The listing builds one solid part. Answer for the finished solid, in the listing's coordinates (mm). Face numbers are marked on the shaded views. A direction names the side the tool comes from. Round coordinates to 2 decimals unless told otherwise and drop trailing zeros. Write each loop counter-clockwise with the first axis right and the second up, starting at its lowest first coordinate (ties: lowest second). Pieces come first, ordered by that corner, then holes.
(1) Each of these flat-tipped pins is pushed along its axis until it touches: pin 1 Ø3.5 at (y, z) = (14, 1) entering from +X; pin 2 Ø3.5 at (y, z) = (-2, 1) entering from -X; pin 3 Ø3 at (y, z) = (8, 10.5) entering from -X; pin 4 Ø5 at (x, y) = (0, 8.5) entering from -Z. Where does it stop, or does it pass through?
(2) For the marked faces 1 and 2, determine the directions among +Z, -Z, +X, -X, +Y, -Y from which every point of the face is accessible in a straight line to the end or side of a thin tool.
(3) The mould has two halves that part along Y. Classify the marked faces 3, 4 and 5: +Y half, -Y half, draft (parallel to the pull), parting line (faces both ways), or undercut.
(4) A cutting plane is placed at A-A, the plane y = 0. Give the vertices of the cut face in (x, z) (3 decimals).
(5) A cutting plane is placed at C-C, the plane z = 10.25. Give the vertices of the cut face in (x, y) (3 decimals), and give its area (3 significant figures).
(6) Find the intervals of material crossed by probe 1 along Y at (x, z) = (0, 1.75) (3 decimals); probe 2 along Y at (x, z) = (-15, 3) (3 decimals); probe 3 along Y at (x, z) = (4.5, 2.5) (3 decimals), in increasing order.
(7) A cutting plane is placed at B-B, the plane x = 0. Give the vertices of the cut face in (y, z) (3 decimals).
from build123d import *

# Parameters (mm, degrees)
F0_R     = 21.125
F1_DEPTH = 21.83
F2_SIZE  = 4.7498
F3_R     = 20.5562247393
F3_W     = 13
F3_H     = 8
F4_DEPTH = 3.175
F5_W     = 12.1872002035
F5_H     = 7.1872002035
F5_R     = 3.1168821316
F6_DEPTH = 1.27


with BuildPart() as f1:
    # F0 (on Top) → F1 (new body)
    with BuildSketch(Plane.XY):
        Circle(F0_R)
    extrude(amount=F1_DEPTH)

    # F2
    f2_edges = [f1.edges().sort_by_distance(p)[0] for p in [
        (-21.125, 0, 21.83),
    ]]
    chamfer(f2_edges, length=F2_SIZE)

    # F3 (on face) → F4 (cut)
    with BuildSketch(Plane(origin=(0, 0, 0), x_dir=(1, 0, 0), z_dir=(0, 0, -1))):
        Circle(F3_R)
        with BuildLine():
            ThreePointArc((3.2638985791, -9.8780455391), (0.0405954465, -13.138647533), (-3.2628129974, -9.9592291742))
            Line((-3.2628129974, -9.9592291742), (-3.2628129974, -19.0050496832))
            ThreePointArc((-3.2628129974, -19.0050496832), (-0.0005507347, 19.2830978272), (3.2638985791, -19.0048632772))
            Line((3.2638985791, -19.0048632772), (3.2638985791, -9.8780455391))
        make_face(mode=Mode.SUBTRACT)
        with Locations((3.625, -0.125)):
            Rectangle(F3_W, F3_H)
        with BuildLine():
            ThreePointArc((3.2638985791, -9.8780455391), (3.2638996448, -9.8765227697), (3.2639, -9.875))
            ThreePointArc((3.2639, -9.875), (-0.042118094, -6.611371762), (-3.2628129974, -9.9592291742))
            ThreePointArc((-3.2628129974, -9.9592291742), (0.0405954465, -13.138647533), (3.2638985791, -9.8780455391))
        make_face()
    extrude(amount=-F4_DEPTH, mode=Mode.SUBTRACT)

    # F5 (on face) → F6 (join)
    with BuildSketch(Plane(origin=(0, 0, 3.175), x_dir=(1, 0, 0), z_dir=(0, 0, -1))):
        with Locations((3.625, -0.125)):
            Rectangle(F5_W, F5_H)
        with Locations((-0.0405954465, -9.8780455391)):
            Circle(F5_R)
    extrude(amount=F6_DEPTH)


solid = f1.part
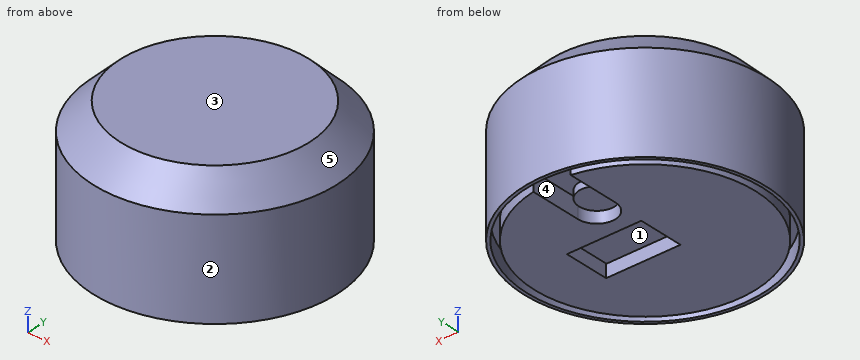
Solutions:
1. pin 1: stops at x = 17.21
1. pin 2: stops at x = -21.12
1. pin 3: stops at x = -20.1
1. pin 4: stops at z = 0
2. face 1: -Z
2. face 2: +Z, -Z
3. face 3: draft
3. face 4: undercut
3. face 5: parting line
4. outline: (-21.125, 0) - (-20.556, 0) - (-20.556, 3.175) - (-19.283, 3.175) - (-19.283, 0) - (-2.875, 0) - (-2.875, 3.175) - (-2.469, 3.175) - (-2.469, 1.905) - (9.719, 1.905) - (9.719, 3.175) - (10.125, 3.175) - (10.125, 0) - (19.283, 0) - (19.283, 3.175) - (20.556, 3.175) - (20.556, 0) - (21.125, 0) - (21.125, 17.08) - (16.375, 21.83) - (-16.375, 21.83) - (-21.125, 17.08) - close
5. outline: circle Ø42.25 at (0, 0)
5. area: 1,400 mm2
6. probe 1: y = -21.125 to -20.556, -19.283 to -3.875, 4.125 to 6.611, 20.556 to 21.125
6. probe 2: y = -14.875 to -14.056, -12.118 to 12.118, 14.056 to 14.875
6. probe 3: y = -20.64 to -20.058, -18.751 to -3.875, -3.469 to 3.719, 4.125 to 18.751, 20.058 to 20.64
7. outline: (-21.125, 0) - (-20.556, 0) - (-20.556, 3.175) - (-19.283, 3.175) - (-19.283, 0) - (-3.875, 0) - (-3.875, 3.175) - (-3.469, 3.175) - (-3.469, 1.905) - (3.719, 1.905) - (3.719, 3.175) - (4.125, 3.175) - (4.125, 0) - (6.611, 0) - (6.611, 3.175) - (6.761, 3.175) - (6.761, 1.905) - (12.995, 1.905) - (12.995, 3.175) - (20.556, 3.175) - (20.556, 0) - (21.125, 0) - (21.125, 17.08) - (16.375, 21.83) - (-16.375, 21.83) - (-21.125, 17.08) - close
